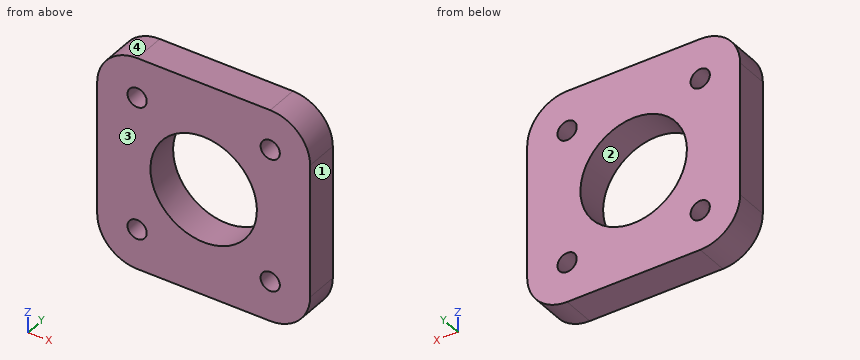
from build123d import *

# Parameters (mm, degrees)
SKETCH1_R           = 8
SKETCH1_R_2         = 1.445711851
BOSS_EXTRUDE1_DEPTH = 5


with BuildPart() as part:
    # Sketch1 → Boss-Extrude1 (new body)
    with BuildSketch(Plane(origin=(0, 0, 0), x_dir=(1, 0, 0), z_dir=(0, 1, 0))):
        with BuildLine():
            Line((-10, 16), (10, 16))
            ThreePointArc((10, 16), (14.242640687, 14.242640687), (16, 10))
            Line((16, 10), (16, -10))
            ThreePointArc((16, -10), (14.242640687, -14.242640687), (10, -16))
            Line((10, -16), (-10, -16))
            ThreePointArc((-10, -16), (-14.242640687, -14.242640687), (-16, -10))
            Line((-16, -10), (-16, 10))
            ThreePointArc((-16, 10), (-14.242640687, 14.242640687), (-10, 16))
        make_face()
        with Locations(Location((0, 0, 0), (0, 0, 270))):
            Circle(SKETCH1_R, mode=Mode.SUBTRACT)
        with Locations(Location((-10, 10, 0), (0, 0, 270))):
            Circle(SKETCH1_R_2, mode=Mode.SUBTRACT)
        with Locations(Location((10, 10, 0), (0, 0, 270))):
            Circle(SKETCH1_R_2, mode=Mode.SUBTRACT)
        with Locations(Location((10, -10, 0), (0, 0, 270))):
            Circle(SKETCH1_R_2, mode=Mode.SUBTRACT)
        with Locations(Location((-10, -10, 0), (0, 0, 270))):
            Circle(SKETCH1_R_2, mode=Mode.SUBTRACT)
    extrude(amount=-BOSS_EXTRUDE1_DEPTH)


solid = part.part
Can you work these out from the model? Positions are in its coordinate system, mm. Face numbers are marked on the shaded views. Give positions to 0.01 mm unless a question says otherwise; leave off trailing zeros. Loops run counter-clockwise (first coordinate to the right, second up) from the corner with the lowest first, then second, coordinate; pieces in that order, holes last. Notation, with made-up numbers: (70.25, 38) -> (95.25, 38) arc R26 ccw to (95.25, 60) -> close; hole circle Ø3 at (22, -36.5). An arc over 180 degrees is marked (long way). Use one line per item in the form item = value.
1) I need wall thicknesses on line 1 along X through (y, z) = (-1.7, -10); line 2 along Z through (x, y) = (-11, -0.6); line 3 along X through (y, z) = (-3.85, 5) (3 decimals). Which ranges of each line are inside material? Lowest first, please.
Answers:
line_1 = -16 to -11.45, -8.55 to 8.55, 11.45 to 16
line_2 = -15.92 to -11.04, -8.96 to 8.96, 11.04 to 15.92
line_3 = -16 to -6.245, 6.245 to 16
2) If we section it at D-D (z = 10.5): Please give me the cut outline in (x, y), plus the area to 3 significant figures.
Answers:
outline = (-15.98, -5) -> (-11.36, -5) -> (-11.36, 0) -> (-15.98, 0) -> close; (-8.64, -5) -> (8.64, -5) -> (8.64, 0) -> (-8.64, 0) -> close; (11.36, -5) -> (15.98, -5) -> (15.98, 0) -> (11.36, 0) -> close
area = 133 mm²
3) If we section it at B-B (y = -1.05): Please give me the cut outline in (x, z).
Answers:
outline = (-16, -10) arc R6 ccw to (-10, -16) -> (10, -16) arc R6 ccw to (16, -10) -> (16, 10) arc R6 ccw to (10, 16) -> (-10, 16) arc R6 ccw to (-16, 10) -> close; hole circle Ø2.89 at (-10, -10); hole circle Ø2.89 at (-10, 10); hole circle Ø16 at (0, 0); hole circle Ø2.89 at (10, -10); hole circle Ø2.89 at (10, 10)
4) Will these pins go through, and if not, where does the flat tip stop? pin 1 (1 mm diameter, centred on x = -13, y = -1, fed in from -Z); pin 2 (1 mm diameter, centred on x = 12.5, y = -4.5, fed in from +Z).
Answers:
pin_1 = -15.45
pin_2 = 15.66
5) We'd pull the mould along X, two halves only. Please class the marked faces 1, 2, 3 and 4: released by +X, released by -X, zero draft, split by the parting line, or undercut.
Answers:
face_1 = released by +X
face_2 = undercut
face_3 = zero draft
face_4 = released by -X
6) If we section it at C-C (z = 0): Please give me the cut outline in (x, y).
Answers:
outline = (-16, -5) -> (-8, -5) -> (-8, 0) -> (-16, 0) -> close; (8, -5) -> (16, -5) -> (16, 0) -> (8, 0) -> close
7) If we section it at A-A (x = 0): Please give me the cut outline in (y, z), plus the area to 3 significant figures.
Answers:
outline = (-5, -16) -> (0, -16) -> (0, -8) -> (-5, -8) -> close; (-5, 8) -> (0, 8) -> (0, 16) -> (-5, 16) -> close
area = 80.0 mm²
